For this review, use the dimensioned drawing (mm, ordinates from the lowest corner) and the shaded views. Coordinates: 2 decimals unless noted, no trailing zeros. Order: outer loops, then holes, each group sorted by start corner. A loop starts at its lowest first (then second) coordinate and runs counter-clockwise, first axis right, second up. Notation, with made-up numbers: M 75.25,46.5 L 85.25,46.5 A31 ccw 85.25,80.5 Z; hole C 11,53.25 d11. An arc over 180 degrees is marked long. Write each question's results on one line, items separated by ' | '.
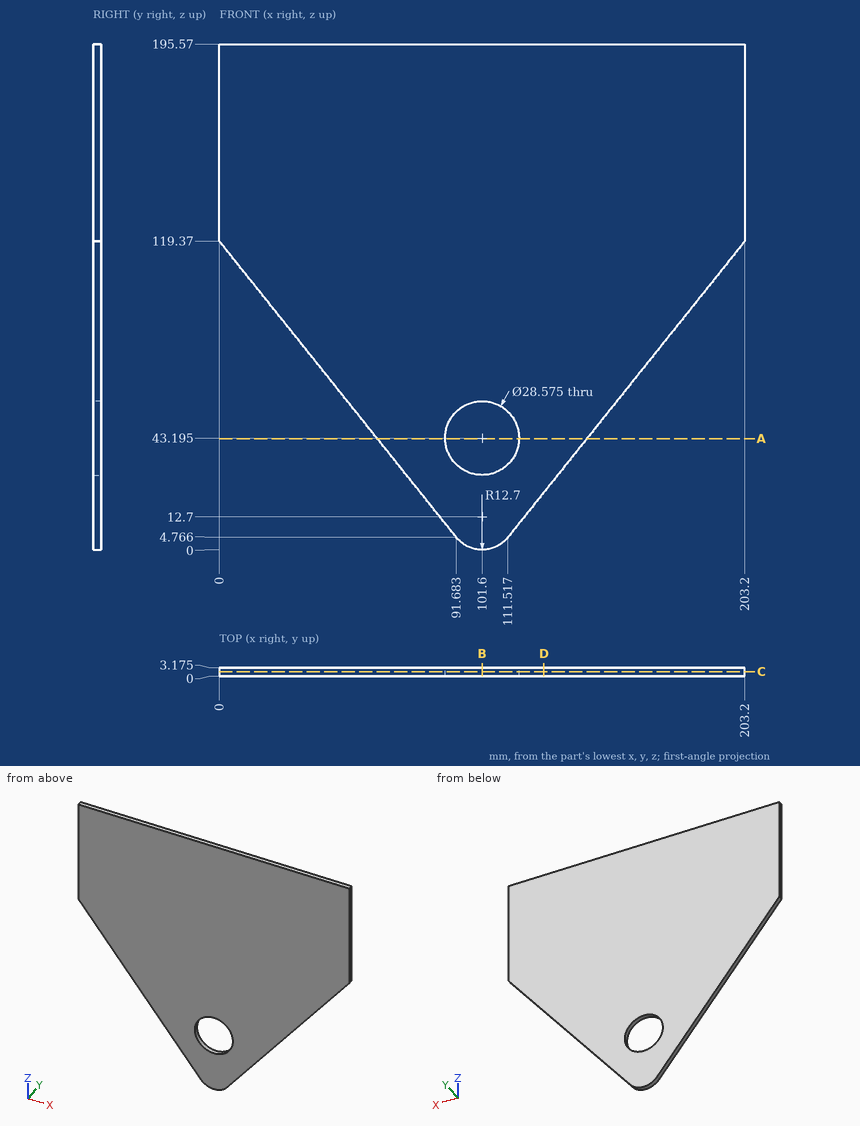
1) For pin 1 (1 mm diameter, centred on y = 1, z = 28, fed in from -X) (1 decimal); pin 2 (8 mm diameter, centred on x = 94, z = 36, fed in from +Y) (3 decimals), all flat-tipped, find the tip position at first contact; note any pin that passes through.
Solutions:
pin 1: x = 72.7 | pin 2: y = 3.175
2) Take a section at B-B on x = 101.6. State the section outline as (y, z) points (1 decimal), plus the area to 3 significant figures.
Solutions:
outline: M 0,0 L 3.2,0 L 3.2,28.9 L 0,28.9 Z; M 0,57.5 L 3.2,57.5 L 3.2,195.6 L 0,195.6 Z | area: 530 mm2
3) To check wall thickness, follow line 1 along Z through (x, y) = (91.5, 1.8) (1 decimal); line 2 along X through (y, z) = (0.9, 46) (1 decimal); line 3 along Z through (x, y) = (85, 0.5). State the ranges of each line that lie inside material, in increasing order.
Solutions:
line 1: 5 to 33.1, 53.3 to 195.6 | line 2: 58.7 to 87.6, 115.6 to 144.5 | line 3: 13.12 to 195.57
4) Take a section at C-C on y = 1.7. State the section outline as (x, z) points (1 decimal), plus the area to 3 significant figures.
Solutions:
outline: M 0,119.4 L 91.7,4.8 A12.7 ccw 111.5,4.8 L 203.2,119.4 L 203.2,195.6 L 0,195.6 Z; hole C 101.6,43.2 d28.6 | area: 27,700 mm2
5) Take a section at A-A on z = 43. State the section outline as (x, y) points (1 decimal).
Solutions:
outline: M 61.1,0 L 87.3,0 L 87.3,3.2 L 61.1,3.2 Z; M 115.9,0 L 142.1,0 L 142.1,3.2 L 115.9,3.2 Z
6) Take a section at D-D on x = 125.5. State the section outline as (y, z) points (1 decimal).
Solutions:
outline: M 0,22.2 L 3.2,22.2 L 3.2,195.6 L 0,195.6 Z
